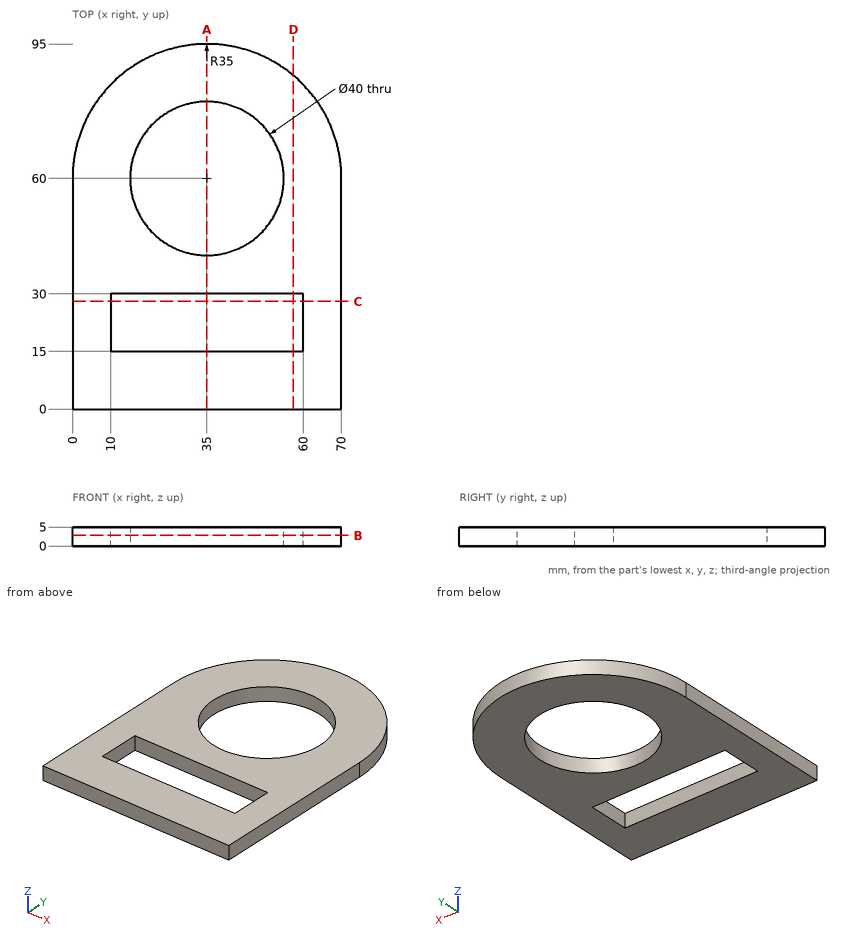
Study the drawing (mm; zero at the part's minimum x, y, z) and answer. Give positions to 0.01 mm unless a question says otherwise; leave off trailing zeros. Order: outer loops, then holes, each group sorted by start corner. A loop starts at its lowest first (then second) coordinate and runs counter-clockwise, first axis right, second up.
1. Straight lines are drawn through the part: L1, parallel to Y at x = 35, z = 1.4; L2, parallel to X at y = 21.5, z = 4.5; L3, parallel to Y at x = 19.5, z = 3.85. For each, find the intervals that lie inside material, in ascending order.
Result sheet:
L1: y = 0 to 15, 30 to 40, 80 to 95
L2: x = 0 to 10, 60 to 70
L3: y = 0 to 15, 30 to 47.36, 72.64 to 91.38
2. Section C-C, the plane y = 28 is taken. Determine the outline of the cut face in (x, z), and give its area (3 significant figures).
Result sheet:
outline: (0, 0) - (10, 0) - (10, 5) - (0, 5) - close; (60, 0) - (70, 0) - (70, 5) - (60, 5) - close
area: 100 mm2
3. Section A-A, the plane x = 35 is taken. Determine the outline of the cut face in (y, z).
Result sheet:
outline: (0, 0) - (15, 0) - (15, 5) - (0, 5) - close; (30, 0) - (40, 0) - (40, 5) - (30, 5) - close; (80, 0) - (95, 0) - (95, 5) - (80, 5) - close
4. This flat-tipped pin is pushed along its axis until it touches: P1, Ø1.5, axis at x = 44.5, z = 1.5, coming from the +Y side. Where does it stop, or does it pass through?
Result sheet:
P1: stops at y = 93.89
5. Section B-B, the plane z = 2.8 is taken. Determine the outline of the cut face in (x, y).
Result sheet:
outline: (0, 0) - (70, 0) - (70, 60) arc R35 ccw to (0, 60) - close; hole (10, 15) - (60, 15) - (60, 30) - (10, 30) - close; hole circle Ø40 at (35, 60)
6. Section D-D, the plane x = 57.5 is taken. Determine the outline of the cut face in (y, z), and give its area (3 significant figures).
Result sheet:
outline: (0, 0) - (15, 0) - (15, 5) - (0, 5) - close; (30, 0) - (86.81, 0) - (86.81, 5) - (30, 5) - close
area: 359 mm2
